Source: CAD feature listing. Evaluate the final solid. Frame: model axes, mm. A direction names the side the tool comes from. Round coordinates to 2 decimals unless told otherwise and drop trailing zeros. Loops run counter-clockwise (first coordinate to the right, second up) from the corner with the lowest first, then second, coordinate; pieces in that order, holes last. Notation, with made-up numbers: M 42.5,42 L 56.5,42 A32 ccw 56.5,72 Z; hole C 63.25,35 d11. An arc over 180 degrees is marked long. Write each question's results on one line, items separated by ' | '. Start each with the question number.
1. Section C-C on y = 25. Output: boundary loops of the cut face in (x, z).
2. Section B-B on x = 18.5. Output: boundary loops of the cut face in (y, z), and give its area (3 significant figures).
3. Set-up query: faces 1 (the flat face through (23, 13, 9.5)), 2 (the flat face through (12, 4, 9)), 3 (the flat face through (12, 2, 11)), 4 (the flat face through (21, 13, 8)), 5 (the flat face through (7, 25, 9)). Return all of +Z, -Z, +X, -X, +Y, -Y with unobstructed straight access to the full face (end or side cutting, diameter ignored); none if empty.
4. Ray query, line 1 (Y direction, x = 2, z = 9.15); line 2 (X direction, y = 2, z = 9.75); line 3 (Y direction, x = 2, z = 9.55). Return the intervals inside material, ascending.
5. Draft query along Y for faces 6 (the cylindrical face through (23, 24, 9)), 7 (the flat face through (3, 27, 9)), 8 (the flat face through (21, 25, 11)), 9 (the cylindrical face through (24, 2, 9)). Return one class per face: released by +Y, released by -Y, zero draft, split by the parting line, or undercut.
6. Contact query for flat-ended pins moving along their axis: pin 1 Ø1.5 at (x, z) = (15.5, 8.5) entering from +Y; pin 2 Ø4.5 at (x, y) = (23.5, 11) entering from +Z. Output: stop coordinate, or through.
7. Section A-A on z = 10.5. Output: boundary loops of the cut face in (x, y), and give its area (3 significant figures).
8. Section D-D on y = 2. Output: boundary loops of the cut face in (x, z), and give its area (3 significant figures).
from build123d import *

# Parameters (mm, degrees)
RECTANGLE_W      = 25
RECTANGLE_H      = 27
EXTRUDE008_DEPTH = 7
RECTANGLE003_W   = 26
RECTANGLE003_H   = 18
EXTRUDE007_DEPTH = 1.5
RECTANGLE002_W   = 11
RECTANGLE002_H   = 5
EXTRUDE006_DEPTH = 11
CIRCLE002_R      = 1
EXTRUDE004_DEPTH = 11
CIRCLE003_R      = 1
EXTRUDE005_DEPTH = 11
CIRCLE001_R      = 1
EXTRUDE003_DEPTH = 11
CIRCLE_R         = 1
EXTRUDE002_DEPTH = 11
RECTANGLE001_W   = 17
RECTANGLE001_H   = 19
EXTRUDE001_DEPTH = 11
EXTRUDE_DEPTH    = 11


with BuildPart() as smaller:
    # Rectangle → Extrude008 (new body)
    with BuildSketch(Plane.XY):
        with Locations((12.5, 13.5)):
            Rectangle(RECTANGLE_W, RECTANGLE_H)
    extrude(amount=EXTRUDE008_DEPTH)


with BuildPart() as extrude007:
    # Rectangle003 → Extrude007 (new body)
    with BuildSketch(Plane(origin=(0, 4, 9.5), x_dir=(1, 0, 0), z_dir=(0, 0, 1))):
        with Locations((13, 9)):
            Rectangle(RECTANGLE003_W, RECTANGLE003_H)
    extrude(amount=EXTRUDE007_DEPTH)


with BuildPart() as extrude006:
    # Rectangle002 → Extrude006 (new body)
    with BuildSketch(Plane(origin=(7, 22, 0), x_dir=(1, 0, 0), z_dir=(0, 0, 1))):
        with Locations((5.5, 2.5)):
            Rectangle(RECTANGLE002_W, RECTANGLE002_H)
    extrude(amount=EXTRUDE006_DEPTH)


with BuildPart() as obj1:
    # Circle002 → Extrude004 (new body)
    with BuildSketch(Plane(origin=(2, 2, 0), x_dir=(1, 0, 0), z_dir=(0, 0, 1))):
        Circle(CIRCLE002_R)
    extrude(amount=EXTRUDE004_DEPTH)


with BuildPart() as obj2:
    # Circle003 → Extrude005 (new body)
    with BuildSketch(Plane(origin=(23, 2, 0), x_dir=(1, 0, 0), z_dir=(0, 0, 1))):
        Circle(CIRCLE003_R)
    extrude(amount=EXTRUDE005_DEPTH)


with BuildPart() as obj3:
    # Circle001 → Extrude003 (new body)
    with BuildSketch(Plane(origin=(23, 25, 0), x_dir=(1, 0, 0), z_dir=(0, 0, 1))):
        Circle(CIRCLE001_R)
    extrude(amount=EXTRUDE003_DEPTH)


with BuildPart() as obj4:
    # Circle → Extrude002 (new body)
    with BuildSketch(Plane(origin=(2, 25, 0), x_dir=(1, 0, 0), z_dir=(0, 0, 1))):
        Circle(CIRCLE_R)
    extrude(amount=EXTRUDE002_DEPTH)


with BuildPart() as extrude_inner:
    # Rectangle001 → Extrude001 (new body)
    with BuildSketch(Plane(origin=(4, 4, 0), x_dir=(1, 0, 0), z_dir=(0, 0, 1))):
        with Locations((8.5, 9.5)):
            Rectangle(RECTANGLE001_W, RECTANGLE001_H)
    extrude(amount=EXTRUDE001_DEPTH)


with BuildPart() as cut007:
    # Rectangle → Extrude (new body)
    with BuildSketch(Plane.XY):
        with Locations((12.5, 13.5)):
            Rectangle(RECTANGLE_W, RECTANGLE_H)
    extrude(amount=EXTRUDE_DEPTH)

    # Cut: cut Extrude inner
    add(extrude_inner.part, mode=Mode.SUBTRACT)

    # Cut001: cut obj4
    add(obj4.part, mode=Mode.SUBTRACT)

    # Cut002: cut obj3
    add(obj3.part, mode=Mode.SUBTRACT)

    # Cut003: cut obj2
    add(obj2.part, mode=Mode.SUBTRACT)

    # Cut004: cut obj1
    add(obj1.part, mode=Mode.SUBTRACT)

    # Cut005: cut Extrude006
    add(extrude006.part, mode=Mode.SUBTRACT)

    # Cut006: cut Extrude007
    add(extrude007.part, mode=Mode.SUBTRACT)

    # Cut007: cut smaller
    add(smaller.part, mode=Mode.SUBTRACT)


solid = cut007.part
Taken from the geometry:
1) outline: M 0,7 L 1,7 L 1,11 L 0,11 Z; M 3,7 L 7,7 L 7,11 L 3,11 Z; M 18,7 L 22,7 L 22,11 L 18,11 Z; M 24,7 L 25,7 L 25,11 L 24,11 Z
2) outline: M 0,7 L 4,7 L 4,11 L 0,11 Z; M 23,7 L 27,7 L 27,11 L 23,11 Z | area: 32.0 mm^2
3) face 1: +Z, +X, -X | face 2: +Z | face 3: +Z, +X, -X, +Y, -Y | face 4: +Z, -Z | face 5: +Z, -Z, +Y
4) line 1: 0 to 1, 3 to 24, 26 to 27 | line 2: 0 to 1, 3 to 22, 24 to 25 | line 3: 0 to 1, 3 to 4, 22 to 24, 26 to 27
5) face 6: undercut | face 7: released by +Y | face 8: zero draft | face 9: undercut
6) pin 1: y = 4 | pin 2: z = 9.5
7) outline: M 0,0 L 25,0 L 25,4 L 0,4 Z; M 0,22 L 4,22 L 4,23 L 7,23 L 7,27 L 0,27 Z; M 18,23 L 21,23 L 21,22 L 25,22 L 25,27 L 18,27 Z; hole C 2,2 d2; hole C 2,25 d2; hole C 23,2 d2; hole C 23,25 d2 | area: 151 mm^2
8) outline: M 0,7 L 1,7 L 1,11 L 0,11 Z; M 3,7 L 22,7 L 22,11 L 3,11 Z; M 24,7 L 25,7 L 25,11 L 24,11 Z | area: 84.0 mm^2
